Source: CAD feature listing. Evaluate the final solid. Frame: model axes, mm. Round coordinates to 2 decimals unless told otherwise and drop trailing zeros. Order: outer loops, then holes, each group sorted by start corner. A loop starts at its lowest first (then second) coordinate and runs counter-clockwise, first axis right, second up. Notation, with made-up numbers: (55, -18) -> (90, -18) arc R7 cw to (90, -8) -> close; hole circle Ø2 at (18, 80.25). An arc over 180 degrees is marked (long way). Use a Markdown table: item, result. Add a question column.
```python
from build123d import *

# Parameters (mm, degrees)
SKETCH1_R           = 11
SKETCH1_R_2         = 1.75
BOSS_EXTRUDE1_DEPTH = 5


with BuildPart() as part:
    # Sketch1 → Boss-Extrude1 (new body)
    with BuildSketch(Plane.XY):
        with BuildLine():
            Line((-14.617184106, 23.367184106), (-20, 0))
            Line((-20, 0), (-20, -20))
            Line((-20, -20), (20, -20))
            Line((20, -20), (20, 0))
            Line((20, 0), (14.617184106, 23.367184106))
            ThreePointArc((14.617184106, 23.367184106), (0, 35), (-14.617184106, 23.367184106))
        make_face()
        with Locations((0, 20)):
            Circle(SKETCH1_R, mode=Mode.SUBTRACT)
        with Locations((-15, -10)):
            Circle(SKETCH1_R_2, mode=Mode.SUBTRACT)
        with Locations((15, -10)):
            Circle(SKETCH1_R_2, mode=Mode.SUBTRACT)
    extrude(amount=BOSS_EXTRUDE1_DEPTH)


solid = part.part
```
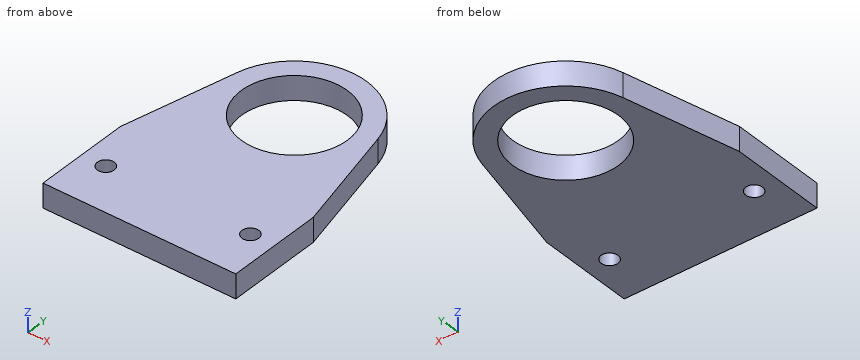
1) First-contact query: pin 1 Ø4.5 at (x, y) = (-15, -10) entering from +Z; pin 2 Ø3 at (x, z) = (7, 1.5) entering from +Y; pin 3 Ø3 at (y, z) = (7, 2) entering from +X. Flat tips, straight axial feed; report the tip coordinate or a pass-through.
2) Line query: probe 1 along Y at (x, z) = (0, 1.2); probe 2 along Y at (x, z) = (8, 0.95); probe 3 along X at (y, z) = (27.5, 0.4). Output: solid intervals per line, ascending. Write a range as from..to.
3) Section C-C on y = 20. Output: boundary loops of the cut face in (x, z).
4) Section B-B on x = 0. Output: boundary loops of the cut face in (y, z), then the cut area to 3 significant figures.
5) Section A-A on z = 1.75. Output: boundary loops of the cut face in (x, y), then the cut area to 3 significant figures.
Conclusion:
| question | item | result |
|---|---|---|
| 1 | pin 1 | stops at z = 5 |
| 1 | pin 2 | stops at y = 33.96 |
| 1 | pin 3 | stops at x = 18.73 |
| 2 | probe 1 | y = -20..9, 31..35 |
| 2 | probe 2 | y = -20..12.45, 27.55..32.69 |
| 2 | probe 3 | x = -12.99..-8.05, 8.05..12.99 |
| 3 | outline | (-15.39, 0) -> (-11, 0) -> (-11, 5) -> (-15.39, 5) -> close; (11, 0) -> (15.39, 0) -> (15.39, 5) -> (11, 5) -> close |
| 4 | outline | (-20, 0) -> (9, 0) -> (9, 5) -> (-20, 5) -> close; (31, 0) -> (35, 0) -> (35, 5) -> (31, 5) -> close |
| 4 | area | 165 mm^2 |
| 5 | outline | (-20, -20) -> (20, -20) -> (20, 0) -> (14.62, 23.37) arc R15 ccw to (-14.62, 23.37) -> (-20, 0) -> close; hole circle Ø3.5 at (-15, -10); hole circle Ø22 at (0, 20); hole circle Ø3.5 at (15, -10) |
| 5 | area | 1,460 mm^2 |
